Source: CAD feature listing. Evaluate the final solid. Frame: model axes, mm. Face numbers are marked on the shaded views. Coordinates: 2 decimals unless noted, no trailing zeros. Loops run counter-clockwise (first coordinate to the right, second up) from the corner with the lowest first, then second, coordinate; pieces in that order, holes last. Notation, with made-up numbers: (76.5, 38) - (113.5, 38) arc R29 ccw to (113.5, 60) - close; hole circle Ø1 at (41.25, 65.25). An arc over 180 degrees is marked (long way). Use one line per item in the form item = value. Start each with the question number.
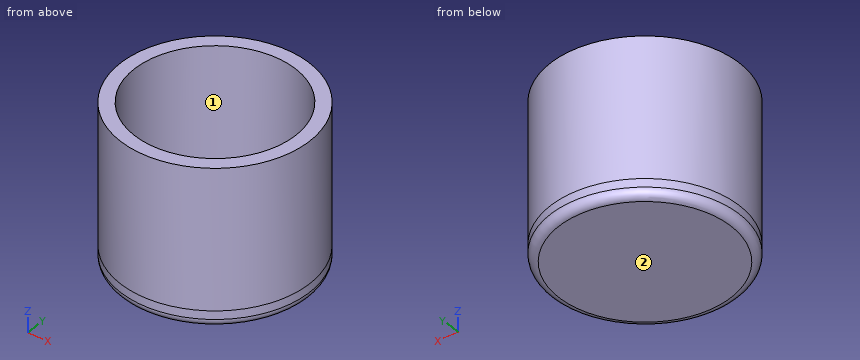
from build123d import *

# Parameters (mm, degrees)
SKETCH1_R           = 16.95
SKETCH1_R_2         = 14.45
BOSS_EXTRUDE1_DEPTH = 25
SKETCH2_R           = 16.95
BOSS_EXTRUDE2_DEPTH = 3
FILLET1_R           = 1.5


with BuildPart() as part:
    # Sketch1 → Boss-Extrude1 (new body)
    with BuildSketch(Plane.XY):
        Circle(SKETCH1_R)
        Circle(SKETCH1_R_2, mode=Mode.SUBTRACT)
    extrude(amount=BOSS_EXTRUDE1_DEPTH)

    # Sketch2 → Boss-Extrude2 (add)
    with BuildSketch(Plane(origin=(0, 0, 0), x_dir=(-1, 0, 0), z_dir=(0, 0, -1))):
        Circle(SKETCH2_R)
    extrude(amount=BOSS_EXTRUDE2_DEPTH)

    # Fillet1
    fillet1_edges = [part.edges().sort_by_distance(p)[0] for p in [
        (16.95, 0, -3),
    ]]
    fillet(fillet1_edges, radius=FILLET1_R)


solid = part.part
(1) Cut plane A-A, the plane y = 0. Output: boundary loops of the cut face in (x, z).
(2) Contact query for flat-ended pins moving along their axis: pin 1 (5 mm diameter, centred on x = -6, z = 16, fed in from -Y); pin 2 (6 mm diameter, centred on x = 6.5, y = 3.5, fed in from +Z); pin 3 (8 mm diameter, centred on y = -6, z = 18, fed in from +X). Output: stop coordinate, or through.
(3) Mould query, pull axis Y, two halves, no side actions, for the marked faces 1 and 2. Classes: +Y half, -Y half, draft (parallel to the pull), parting line (faces both ways), or undercut.
(4) Cut plane C-C, the plane z = 10. Output: boundary loops of the cut face in (x, y), plus the area to 3 significant figures.
(5) Material intervals for line 1 (Y direction, x = 0, z = 5); line 2 (Z direction, x = 3, y = 9); line 3 (Y direction, x = -4.5, z = 14.5), sorted ascending.
Recorded:
q1.outline = (-16.95, -1.5) arc R1.5 ccw to (-15.45, -3) - (15.45, -3) arc R1.5 ccw to (16.95, -1.5) - (16.95, 25) - (14.45, 25) - (14.45, 0) - (-14.45, 0) - (-14.45, 25) - (-16.95, 25) - close
q2.pin_1 = -16.58
q2.pin_2 = 0
q2.pin_3 = 16.83
q3.face_1 = undercut
q3.face_2 = draft
q4.outline = circle Ø33.9 at (0, 0); hole circle Ø28.9 at (0, 0)
q4.area = 247 mm²
q5.line_1 = -16.95 to -14.45, 14.45 to 16.95
q5.line_2 = -3 to 0
q5.line_3 = -16.34 to -13.73, 13.73 to 16.34
